Geometry check sheet. Reference: the model listing, model coordinates, mm. Give positions to 0.01 mm unless a question says otherwise; leave off trailing zeros. Loops run counter-clockwise (first coordinate to the right, second up) from the corner with the lowest first, then second, coordinate; pieces in that order, holes last. Notation, with made-up numbers: (-18, 79) - (40, 79) arc R9 ccw to (40, 93) - close; hole circle Ø5 at (50.25, 62.5). An arc over 180 degrees is marked (long way). Use a Markdown table: item, result. Add a question column.
1. Depth check by flat-ended pin: P1, Ø2.5, axis at x = -60, z = 0, coming from the +Y side. Enter the tip coordinate at first touch or a pass-through.
2. Material ranges on L1, parallel to X at y = 0.85, z = -0.25; L2, parallel to Z at x = 60, y = 2.1; L3, parallel to X at y = 1.3, z = 1.25, recorded low to high.
3. Cross-section at B-B on x = -60. Enter the section's corners in (y, z).
4. Cross-section at C-C on z = 0. Enter the section's corners in (x, y), and give its area (3 significant figures).
5. Cross-section at A-A on y = 2.8. Enter the section's corners in (x, z), and give its area (3 significant figures).
6. Draft check along X on faces 1 (the cylindrical face through (-61.43, 2.46, -0.45)), 2 (the flat face through (16, 2, 5)), 3 (the flat face through (105, 2, 0)). Enter one of: pulls with the +X half, pulls with the -X half, needs draft (parallel to the pull), parting line crosses it, or undercut.
Autodesk Inventor part; units mm, degrees
ref_plane "YZ Plane" through (0, 0, 0) normal (1, 0, 0) x (0, 1, 0)
ref_plane "XZ Plane" through (0, 0, 0) normal (0, 1, 0) x (-1, 0, 0)
ref_plane "XY Plane" through (0, 0, 0) normal (0, 0, 1) x (1, 0, 0)
sketch "Sketch1" plane through (0, 0, 0) normal (0, 1, 0) x (-1, 0, 0)
  line L0 (70, 5) -> (-70, 5)
  line L1 (-70, -5) -> (70, -5)
  line L2 (70, -5) -> (70, 5)
  line L3 (-70, -5) -> (-105, -5)
  line L4 (-105, -5) -> (-105, 5)
  line L5 (-105, 5) -> (-70, 5)
  circle A0 centre (-78.75, 0) radius 1.5
  circle A1 centre (-96.25, 0) radius 1.5
  circle A2 centre (0, 0) radius 1.5
  circle A3 centre (60, 0) radius 1.5
  circle A4 centre (-60, 0) radius 1.5
extrude "Extrusion1" add sketch "Sketch1" along normal blind 5
properties part number "batang_horn_normal"
Values found:
| question | item | result |
|---|---|---|
| 1 | P1 | passes through |
| 2 | L1 | x = -70 to -61.48, -58.52 to -1.48, 1.48 to 58.52, 61.48 to 77.27, 80.23 to 94.77, 97.73 to 105 |
| 2 | L2 | z = -5 to -1.5, 1.5 to 5 |
| 2 | L3 | x = -70 to -60.83, -59.17 to -0.83, 0.83 to 59.17, 60.83 to 77.92, 79.58 to 95.42, 97.08 to 105 |
| 3 | outline | (0, -5) - (5, -5) - (5, -1.5) - (0, -1.5) - close; (0, 1.5) - (5, 1.5) - (5, 5) - (0, 5) - close |
| 4 | outline | (-70, 0) - (-61.5, 0) - (-61.5, 5) - (-70, 5) - close; (-58.5, 0) - (-1.5, 0) - (-1.5, 5) - (-58.5, 5) - close; (1.5, 0) - (58.5, 0) - (58.5, 5) - (1.5, 5) - close; (61.5, 0) - (77.25, 0) - (77.25, 5) - (61.5, 5) - close; (80.25, 0) - (94.75, 0) - (94.75, 5) - (80.25, 5) - close; (97.75, 0) - (105, 0) - (105, 5) - (97.75, 5) - close |
| 4 | area | 800 mm2 |
| 5 | outline | (-70, -5) - (105, -5) - (105, 5) - (-70, 5) - close; hole circle Ø3 at (-60, 0); hole circle Ø3 at (0, 0); hole circle Ø3 at (60, 0); hole circle Ø3 at (78.75, 0); hole circle Ø3 at (96.25, 0) |
| 5 | area | 1,710 mm2 |
| 6 | face 1 | undercut |
| 6 | face 2 | needs draft |
| 6 | face 3 | pulls with the +X half |
